Read the model definition and answer for the solid it produces. Units are mm, in the model's axes. A direction names the side the tool comes from. Give positions to 0.01 mm unless a question says otherwise; leave off trailing zeros. Write each loop counter-clockwise with the first axis right and the second up, starting at its lowest first coordinate (ties: lowest second). Pieces come first, ordered by that corner, then holes. Notation, with made-up numbers: (63, 5) -> (109, 5) arc R24 ccw to (109, 44) -> close; hole circle Ø8 at (22, -29.75). An arc over 180 degrees is marked (long way). Put each result on its own line as item: value. Start each with the question number.
from build123d import *

# Parameters (mm, degrees)
SKETCH1_W           = 120
SKETCH1_H           = 80
SKETCH1_W_2         = 115.2
SKETCH1_H_2         = 75.2
BOSS_EXTRUDE1_DEPTH = 47.6
SKETCH2_W           = 120
SKETCH2_H           = 80
BOSS_EXTRUDE2_DEPTH = 2.4
SKETCH3_W           = 45
SKETCH3_H           = 45
BOSS_EXTRUDE3_DEPTH = 6
SKETCH4_R           = 1.1
CUT_EXTRUDE1_DEPTH  = 92.301697684
SKETCH5_R           = 1.15
BOSS_EXTRUDE4_DEPTH = 2.5
SKETCH6_R           = 4
SKETCH6_R_2         = 5
CUT_EXTRUDE2_DEPTH  = 3


with BuildPart() as part:
    # Sketch1 → Boss-Extrude1 (new body)
    with BuildSketch(Plane.XY):
        Rectangle(SKETCH1_W, SKETCH1_H)
        Rectangle(SKETCH1_W_2, SKETCH1_H_2, mode=Mode.SUBTRACT)
    extrude(amount=BOSS_EXTRUDE1_DEPTH)

    # Sketch2 → Boss-Extrude2 (add)
    with BuildSketch(Plane.XY.offset(47.6)):
        Rectangle(SKETCH2_W, SKETCH2_H)
    extrude(amount=BOSS_EXTRUDE2_DEPTH)

    # Sketch3 → Boss-Extrude3 (add)
    with BuildSketch(Plane.XY.offset(50)):
        Rectangle(SKETCH3_W, SKETCH3_H)
    extrude(amount=BOSS_EXTRUDE3_DEPTH)

    # Sketch4 → Cut-Extrude1 (cut, through all)
    with BuildSketch(Plane.XY.offset(56)):
        with Locations((-14.1, 14.1)):
            Circle(SKETCH4_R)
        with Locations((14.1, -14.1)):
            Circle(SKETCH4_R)
    extrude(amount=-CUT_EXTRUDE1_DEPTH, mode=Mode.SUBTRACT)

    # Sketch5 → Boss-Extrude4 (add)
    with BuildSketch(Plane.XY.offset(56)):
        with Locations((-15.7, -15.7)):
            Circle(SKETCH5_R)
    extrude(amount=BOSS_EXTRUDE4_DEPTH)

    # Sketch6 → Cut-Extrude2 (cut)
    with BuildSketch(Plane.XY.offset(50)):
        with Locations((-30, -32)):
            Circle(SKETCH6_R)
        with Locations((30, -32)):
            Circle(SKETCH6_R)
        with Locations((0, -30)):
            Circle(SKETCH6_R_2)
    extrude(amount=-CUT_EXTRUDE2_DEPTH, mode=Mode.SUBTRACT)


solid = part.part
1) For a pull along X with two mould halves and no side action, classify faces 5 (the face through (-1.08, -34.88, 48.82)), 6 (the face through (-60, -1, 25)), 7 (the face through (0, 0, 56)) as pulls with the +X half, pulls with the -X half, needs draft (parallel to the pull), parting line crosses it, or undercut.
2) A cutting plane is placed at B-B on z = 46. Give the vertices of the cut face in (x, y), and give its area (3 significant figures).
3) A cutting plane is placed at C-C on y = 35.5. Give the vertices of the cut face in (x, z), and give its area (3 significant figures).
4) Straight lines are drawn through the part: line 1 (Y direction, x = 23, z = 39.5); line 2 (Y direction, x = -14, z = 53); line 3 (X direction, y = 33, z = 11). For each, find the intervals that lie inside material, in ascending order. Write a range as [from, to].
5) For faces 1 (the face through (-22.5, 0, 53)), 2 (the face through (0, 22.5, 53)), 3 (the face through (22.5, 0, 53)), 4 (the face through (-1, 1, 47.6)), determine the directions among +Z, -Z, +X, -X, +Y, -Y from which every point of the face is accessible in a straight line to the end or side of a thin tool.
6) A cutting plane is placed at D-D on y = -32. Give the vertices of the cut face in (x, z), and give its area (3 significant figures).
7) A cutting plane is placed at A-A on x = 30. Give the vertices of the cut face in (y, z), and give its area (3 significant figures).
8) Each of these flat-tipped pins is pushed along its axis until it touches: pin 1 Ø12 at (x, y) = (-22.5, -26) entering from -Z; pin 2 Ø3 at (x, z) = (-3.5, 53) entering from +Y; pin 3 Ø2 at (x, y) = (-14.1, 14.1) entering from -Z; pin 4 Ø22.5 at (x, y) = (9.5, 11) entering from +Z. Where does it stop, or does it pass through?
Results found:
1. face 5: undercut
1. face 6: pulls with the -X half
1. face 7: needs draft
2. outline: (-60, -40) -> (60, -40) -> (60, 40) -> (-60, 40) -> close; hole (-57.6, -37.6) -> (57.6, -37.6) -> (57.6, 37.6) -> (-57.6, 37.6) -> close
2. area: 937 mm²
3. outline: (-60, 0) -> (-57.6, 0) -> (-57.6, 47.6) -> (57.6, 47.6) -> (57.6, 0) -> (60, 0) -> (60, 50) -> (-60, 50) -> close
3. area: 516 mm²
4. line 1: y = [-40, -37.6], [37.6, 40]
4. line 2: y = [-22.5, 13], [15.2, 22.5]
4. line 3: x = [-60, -57.6], [57.6, 60]
5. face 1: +Z, -X, +Y, -Y
5. face 2: +Z, +X, -X, +Y
5. face 3: +Z, +X, +Y, -Y
5. face 4: -Z
6. outline: (-60, 0) -> (-57.6, 0) -> (-57.6, 47.6) -> (-34, 47.6) -> (-34, 50) -> (-60, 50) -> close; (-26, 47.6) -> (-4.58, 47.6) -> (-4.58, 50) -> (-26, 50) -> close; (4.58, 47.6) -> (26, 47.6) -> (26, 50) -> (4.58, 50) -> close; (34, 47.6) -> (57.6, 47.6) -> (57.6, 0) -> (60, 0) -> (60, 50) -> (34, 50) -> close
6. area: 456 mm²
7. outline: (-40, 0) -> (-37.6, 0) -> (-37.6, 47.6) -> (-36, 47.6) -> (-36, 50) -> (-40, 50) -> close; (-28, 47.6) -> (37.6, 47.6) -> (37.6, 0) -> (40, 0) -> (40, 50) -> (-28, 50) -> close
7. area: 401 mm²
8. pin 1: stops at z = 47.6
8. pin 2: stops at y = 22.5
8. pin 3: passes through
8. pin 4: stops at z = 56
